```python
from build123d import *

# Parameters (mm, degrees)
SKETCH_1_W          = 38
SKETCH_1_H          = 34
MIDDLE_PLATE_DEPTH  = 1
MIDDLE_PILLAR_DEPTH = 3
C_CUT_REACH         = 27.807
SKETCH_3_W          = 15
SKETCH_3_H          = 4


with BuildPart() as part:
    # 스케치1 → Middle_plate (new body)
    with BuildSketch(Plane(origin=(0, 0, 0), x_dir=(1, 0, 0), z_dir=(0, 1, 0))):
        Rectangle(SKETCH_1_W, SKETCH_1_H)
    extrude(amount=MIDDLE_PLATE_DEPTH)

    # 스케치2 → Middle_pillar (add)
    with BuildSketch(Plane(origin=(0, 1, 0), x_dir=(1, 0, 0), z_dir=(0, 1, 0))):
        with BuildLine():
            ThreePointArc((17.1, -14), (16.48492424, -12.51507576), (15, -11.9))
            Line((15, -11.9), (15, -12.45))
            ThreePointArc((15, -12.45), (16.096015511, -12.903984489), (16.55, -14))
            ThreePointArc((16.55, -14), (15, -15.55), (13.45, -14))
            Line((13.45, -14), (12.9, -14))
            ThreePointArc((12.9, -14), (15, -16.1), (17.1, -14))
        make_face()
        with BuildLine():
            Line((15, -12.45), (15, -11.9))
            ThreePointArc((15, -11.9), (13.51507576, -12.51507576), (12.9, -14))
            Line((12.9, -14), (13.45, -14))
            ThreePointArc((13.45, -14), (13.903984489, -12.903984489), (15, -12.45))
        make_face()
        with BuildLine():
            ThreePointArc((-15, 12.45), (-16.096015511, 15.096015511), (-13.45, 14))
            Line((-13.45, 14), (-12.9, 14))
            ThreePointArc((-12.9, 14), (-16.48492424, 15.48492424), (-15, 11.9))
            Line((-15, 11.9), (-15, 12.45))
        make_face()
        with BuildLine():
            Line((-12.9, 14), (-13.45, 14))
            ThreePointArc((-13.45, 14), (-13.903984489, 12.903984489), (-15, 12.45))
            Line((-15, 12.45), (-15, 11.9))
            ThreePointArc((-15, 11.9), (-13.51507576, 12.51507576), (-12.9, 14))
        make_face()
    extrude(amount=MIDDLE_PILLAR_DEPTH)

    # 스케치3 → C_cut (cut, up to next)
    with BuildSketch(Plane.XZ, mode=Mode.PRIVATE) as c_cut_sk1:
        with Locations((0, 15)):
            Rectangle(SKETCH_3_W, SKETCH_3_H)
    c_cut_tool1 = extrude(c_cut_sk1.sketch, amount=-C_CUT_REACH, mode=Mode.PRIVATE) & part.part
    add(c_cut_tool1.solids().sort_by_distance((0, 0, 15))[0], mode=Mode.SUBTRACT)


solid = part.part
```
Work out the finished part from the listing and answer in its coordinate system (mm). A direction names the side the tool comes from. Coordinates: 2 decimals unless noted, no trailing zeros. Loops run counter-clockwise (first coordinate to the right, second up) from the corner with the lowest first, then second, coordinate; pieces in that order, holes last. Notation, with made-up numbers: (-35.5, -23) - (8.5, -23) arc R8 ccw to (8.5, -8) - close; hole circle Ø9 at (-4.5, -14). An arc over 180 degrees is marked (long way). Use a Markdown table: item, result.
Item 1: Find section A-A, the plane y = 2.5. Determine the outline of the cut face in (x, z).
Evaluation:
| item | result |
|---|---|
| outline | circle Ø4.2 at (-15, -14); circle Ø4.2 at (15, 14); hole circle Ø3.1 at (-15, -14); hole circle Ø3.1 at (15, 14) |
Item 2: For faces 1 (the flat face through (7.5, 0.5, 15)), 2 (the flat face through (-19, 0.5, 0.2)), determine the directions among +Z, -Z, +X, -X, +Y, -Y from which every point of the face is accessible in a straight line to the end or side of a thin tool.
Evaluation:
| item | result |
|---|---|
| face 1 | +Z, +Y, -Y |
| face 2 | +Z, -Z, -X, +Y, -Y |
Item 3: Given pin 1 Ø2 at (x, z) = (10, 11) entering from +Y; pin 2 Ø0.5 at (x, y) = (0.5, 0.5) entering from +Z; pin 3 Ø2 at (y, z) = (2.5, -3) entering from +X, each flat-ended and moving along its own axis, determine where each tip first touches the part or whether it passes through.
Evaluation:
| item | result |
|---|---|
| pin 1 | stops at y = 1 |
| pin 2 | stops at z = 13 |
| pin 3 | passes through |
Item 4: Consider probe 1 along Z at (x, y) = (-15, 2.25); probe 2 along Y at (x, z) = (-2, -0.5); probe 3 along X at (y, z) = (2.2, -14). Determine where each line is inside the solid, lowest interval first. Write a range as from..to.
Evaluation:
| item | result |
|---|---|
| probe 1 | z = -16.1..-15.55, -12.45..-11.9 |
| probe 2 | y = 0..1 |
| probe 3 | x = -17.1..-16.55, -13.45..-12.9 |
Item 5: Find section D-D, the plane x = 16. Determine the outline of the cut face in (y, z), and give its area (3 significant figures).
Evaluation:
| item | result |
|---|---|
| outline | (0, -17) - (1, -17) - (1, 12.15) - (4, 12.15) - (4, 12.82) - (1, 12.82) - (1, 15.18) - (4, 15.18) - (4, 15.85) - (1, 15.85) - (1, 17) - (0, 17) - close |
| area | 38.0 mm2 |
Item 6: The mould has two halves that part along Z. Classify faces 3 (the flat face through (-0.3, 0.5, -17)), 4 (the flat face through (-15, 1, -14)), 5 (the flat face through (-7.5, 0.5, 15)), 6 (the flat face through (15, 1, 14)): +Z half, -Z half, draft (parallel to the pull), parting line (faces both ways), or undercut.
Evaluation:
| item | result |
|---|---|
| face 3 | -Z half |
| face 4 | undercut |
| face 5 | draft |
| face 6 | undercut |
Item 7: Find section B-B, the plane x = 1.5. Determine the outline of the cut face in (y, z), and give its area (3 significant figures).
Evaluation:
| item | result |
|---|---|
| outline | (0, -17) - (1, -17) - (1, 13) - (0, 13) - close |
| area | 30.0 mm2 |
Item 8: Find section C-C, the plane z = -13. Determine the outline of the cut face in (x, y), and give its area (3 significant figures).
Evaluation:
| item | result |
|---|---|
| outline | (-19, 0) - (19, 0) - (19, 1) - (-13.15, 1) - (-13.15, 4) - (-13.82, 4) - (-13.82, 1) - (-16.18, 1) - (-16.18, 4) - (-16.85, 4) - (-16.85, 1) - (-19, 1) - close |
| area | 42.0 mm2 |
